from build123d import *

# Parameters (mm, degrees)
BOSS_EXTRUDE1_DEPTH     = 25.4
CUT_EXTRUDE1_DEPTH      = 45.012417566
CUT_EXTRUDE1_DEPTH_BACK = 45.012417566
SKETCH2_R               = 3.175
SKETCH3_R               = 6.35
CUT_EXTRUDE3_DEPTH      = 13.97


with BuildPart() as part:
    # Sketch1 → Boss-Extrude1 (new body)
    with BuildSketch(Plane(origin=(0, 0, 0), x_dir=(0, 0, -1), z_dir=(1, 0, 0))):
        with BuildLine():
            Line((27.876340451, 19.05), (30.48, 19.05))
            Line((30.48, 19.05), (30.48, 0))
            Line((30.48, 0), (0, 0))
            Line((0, 0), (0, 19.05))
            Line((0, 19.05), (2.603659549, 19.05))
            ThreePointArc((2.603659549, 19.05), (15.24, 7.62), (27.876340451, 19.05))
        make_face()
    extrude(amount=BOSS_EXTRUDE1_DEPTH)

    # Sketch2 → Cut-Extrude1 (cut, two sides: drawn at the far end of the back side and taken through both)
    with BuildSketch(Plane.XZ.offset(-CUT_EXTRUDE1_DEPTH_BACK)):
        with Locations(Location((12.7, -15.24, 0), (0, 0, 270))):
            Circle(SKETCH2_R)
    extrude(amount=CUT_EXTRUDE1_DEPTH + CUT_EXTRUDE1_DEPTH_BACK, mode=Mode.SUBTRACT)

    # Sketch3 → Cut-Extrude3 (cut)
    with BuildSketch(Plane(origin=(0, 19.05, 0), x_dir=(1, 0, 0), z_dir=(0, 1, 0))):
        with Locations(Location((12.7, 15.24, 0), (0, 0, 270))):
            Circle(SKETCH3_R)
    extrude(amount=-CUT_EXTRUDE3_DEPTH, mode=Mode.SUBTRACT)


solid = part.part
Here's how the part is built. I have some questions about the finished solid (model axes, mm). A direction names the side the tool comes from. Round coordinates to 2 decimals unless told otherwise and drop trailing zeros. Loops run counter-clockwise (first coordinate to the right, second up) from the corner with the lowest first, then second, coordinate; pieces in that order, holes last. Notation, with made-up numbers: M 70,-12.75 L 111,-12.75 A30 cw 111,16.25 Z; hole C -13.75,24 d2. An arc over 180 degrees is marked long. Write each question's results on one line, items separated by ' | '. Start each with the question number.
(1) On a 3-axis mill with a long thin cutter (end or side, diameter ignored), from which of +Z, -Z, +X, -X, +Y, -Y can I reach the whole of each face in a straight line? I mean faces 1 (the flat face through (13, 19.05, -29)), 2 (the cylindrical face through (8.84, 6.76, -20.28)). Say none if no direction works.
(2) I want a section at A-A (y = 16.25). Please give me the cut outline in (x, z).
(3) I want a section at B-B (x = 12.7). Please give me the cut outline in (y, z) (3 decimals).
(4) I want a section at D-D (y = 7). Please give me the cut outline in (x, z).
(5) Will these pins go through, and if not, where does the flat tip stop? P1, Ø3, axis at x = 6, z = -8, coming from the +Y side; P2, Ø3, axis at x = 18.5, z = -13, coming from the +Y side; P3, Ø7.5, axis at x = 12.7, z = -15.24, coming from the +Y side.
(6) If I drill on probe 1 along Z at (x, y) = (12.7, 3.05) (3 decimals); probe 2 along Z at (x, y) = (12.7, 8.4); probe 3 along X at (y, z) = (3.2, -15.24) (3 decimals), over which ranges is the centre line in solid material (lowest first)? Write a range as from..to.
(7) I want a section at C-C (z = -15.24). Please give me the cut outline in (x, y) (3 decimals).
(8) Thinking about a two-plate mould opening in Z: for faces 3 (the flat face through (16, 5.08, -14)), 4 (the flat face through (13, 9, 0)), 5 (the flat face through (13, 0, -19)), 6 (the flat face through (13, 10, -30.48)), which applies, pulls with the +Z half, pulls with the -Z half, needs draft (parallel to the pull), parting line crosses it, or undercut?
Solved:
1) face 1: +Z, -Z, +X, -X, +Y | face 2: +Y
2) outline: M 0,-30.48 L 25.4,-30.48 L 25.4,-27.27 L 0,-27.27 Z; M 0,-3.21 L 25.4,-3.21 L 25.4,0 L 0,0 Z
3) outline: M 0,-30.48 L 19.05,-30.48 L 19.05,-27.876 A12.7 cw 9.321,-21.59 L 5.08,-21.59 L 5.08,-18.415 L 0,-18.415 Z; M 0,-12.065 L 5.08,-12.065 L 5.08,-8.89 L 9.321,-8.89 A12.7 cw 19.05,-2.604 L 19.05,0 L 0,0 Z
4) outline: M 0,-30.48 L 25.4,-30.48 L 25.4,0 L 0,0 Z; hole C 12.7,-15.24 d12.7
5) P1: stops at y = 11.11 | P2: stops at y = 8.18 | P3: stops at y = 5.08
6) probe 1: z = -30.48..-18.415, -12.065..0 | probe 2: z = -30.48..-21.59, -8.89..0 | probe 3: x = 0..9.525, 15.875..25.4
7) outline: M 0,0 L 9.525,0 L 9.525,5.08 L 6.35,5.08 L 6.35,7.62 L 0,7.62 Z; M 15.875,0 L 25.4,0 L 25.4,7.62 L 19.05,7.62 L 19.05,5.08 L 15.875,5.08 Z
8) face 3: undercut | face 4: pulls with the +Z half | face 5: needs draft | face 6: pulls with the -Z half
